Input: part model. Units: mm. Frame: model coordinates. Face numbers are marked on the shaded views. A direction names the side the tool comes from. Give positions to 0.01 mm unless a question says otherwise; leave off trailing zeros. Loops run counter-clockwise (first coordinate to the right, second up) from the corner with the lowest first, then second, coordinate; pieces in that order, holes last.
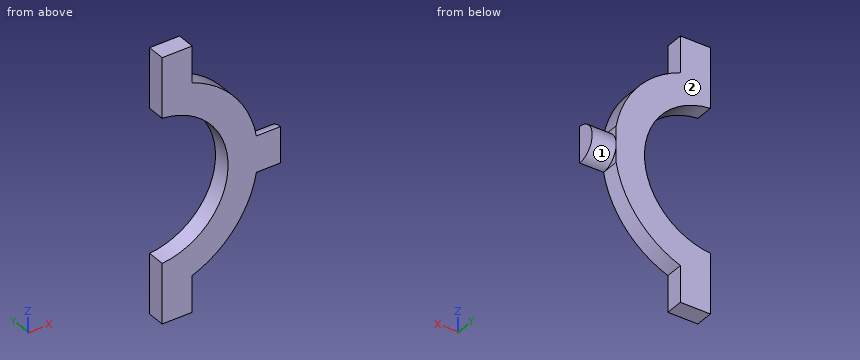
from build123d import *

# Parameters (mm, degrees)
BOSS_EXTRUDE1_DEPTH = 6
SKETCH2_OUTSIDE_W   = 109.13
SKETCH2_OUTSIDE_H   = 27.296
CUT_EXTRUDE1_DEPTH  = 8


with BuildPart() as part:
    # Sketch1 → Boss-Extrude1 (new body)
    with BuildSketch(Plane(origin=(0, 0, 0), x_dir=(1, 0, 0), z_dir=(0, 1, 0))):
        with BuildLine():
            Line((2, 43.916521486), (2, 23.916521486))
            ThreePointArc((2, 23.916521486), (24, 0), (2, -23.916521486))
            Line((2, -23.916521486), (2, -43.916521486))
            Line((2, -43.916521486), (12, -43.916521486))
            Line((12, -43.916521486), (12, -31.811947441))
            ThreePointArc((12, -31.811947441), (26.141204334, -21.740226217), (33.466401061, -6))
            Line((33.466401061, -6), (41.466401061, -6))
            Line((41.466401061, -6), (41.466401061, 6))
            Line((41.466401061, 6), (33.466401061, 6))
            ThreePointArc((33.466401061, 6), (26.141204334, 21.740226217), (12, 31.811947441))
            Line((12, 31.811947441), (12, 43.916521486))
            Line((12, 43.916521486), (2, 43.916521486))
        make_face()
    extrude(amount=BOSS_EXTRUDE1_DEPTH)

    # Sketch2 outside → Cut-Extrude1 (cut)
    with BuildSketch(Plane(origin=(41.466401061, 0, 0), x_dir=(0, 0, -1), z_dir=(1, 0, 0))):
        with Locations((0, 3)):
            Rectangle(SKETCH2_OUTSIDE_W, SKETCH2_OUTSIDE_H)
        with BuildLine():
            Line((-6, 0), (6, 0))
            ThreePointArc((6, 0), (0, 6), (-6, 0))
        make_face(mode=Mode.SUBTRACT)
    extrude(amount=-CUT_EXTRUDE1_DEPTH, mode=Mode.SUBTRACT)


solid = part.part
(1) Cut plane B-B (y = 3.15). Return the cut outline in (x, z), and give its area (3 significant figures).
Values follow:
outline: (2, -43.92) - (12, -43.92) - (12, -31.81) arc R34 ccw to (33.47, -6) - (33.47, -5.11) - (41.47, -5.11) - (41.47, 5.11) - (33.47, 5.11) - (33.47, 6) arc R34 ccw to (12, 31.81) - (12, 43.92) - (2, 43.92) - (2, 23.92) arc R24 cw to (2, -23.92) - close
area: 1,160 mm2
(2) Cut plane C-C (z = -4.5). Return the cut outline in (x, y).
Values follow:
outline: (23.57, 0) - (41.47, 0) - (41.47, 3.97) - (33.47, 3.97) - (33.47, 6) - (23.57, 6) - close
(3) Cut plane D-D (x = 9.5). Return the cut outline in (y, z), and give its area (3 significant figures).
Values follow:
outline: (0, -43.92) - (6, -43.92) - (6, -22.04) - (0, -22.04) - close; (0, 22.04) - (6, 22.04) - (6, 43.92) - (0, 43.92) - close
area: 263 mm2
(4) Ray query, probe 1 along X at (y, z) = (3.95, -37.5); probe 2 along Z at (x, y) = (9.5, 3.7); probe 3 along Z at (x, y) = (13.5, 4.95). Return the intervals inside material, ascending.
Values follow:
probe 1: x = 2 to 12
probe 2: z = -43.92 to -22.04, 22.04 to 43.92
probe 3: z = -31.2 to -19.84, 19.84 to 31.2
(5) Reachability of the marked faces 1 and 2 from +Z, -Z, +X, -X, +Y, -Y: full face, straight path, thin tool, end or side. Return the list, or none.
Values follow:
face 1: +X, +Y
face 2: +Z, -Z, +X, -X, +Y
(6) Cut plane A-A (x = 5.5). Return the cut outline in (y, z), and give its area (3 significant figures).
Values follow:
outline: (0, -43.92) - (6, -43.92) - (6, -23.36) - (0, -23.36) - close; (0, 23.36) - (6, 23.36) - (6, 43.92) - (0, 43.92) - close
area: 247 mm2
(7) Pin query (flat end, axial travel): pin 1 Ø10 at (x, z) = (31.5, 13) entering from +Y; pin 2 Ø1 at (x, y) = (23.5, 4) entering from -Z. Return the tip coordinate at first contact, or that it passes through.
Values follow:
pin 1: stops at y = 6
pin 2: stops at z = -25.04
